Drawing for the job (mm, zero at the part's lowest x, y, z). Round coordinates to 2 decimals unless told otherwise and drop trailing zeros. Write each loop counter-clockwise with the first axis right and the second up, starting at its lowest first coordinate (ties: lowest second). Pieces come first, ordered by that corner, then holes.
Item 1: Wall check: probe 1 along X at (y, z) = (170, 3); probe 2 along Y at (x, z) = (5, 2.1). Give the ranges that are in metal, low to high.
Item 2: Band-saw the part on B-B, the plane x = 5. Write the cut outline in (y, z).
Item 3: Band-saw the part on A-A, the plane y = 5. Write the cut outline in (x, z), then the cut area to 3 significant figures.
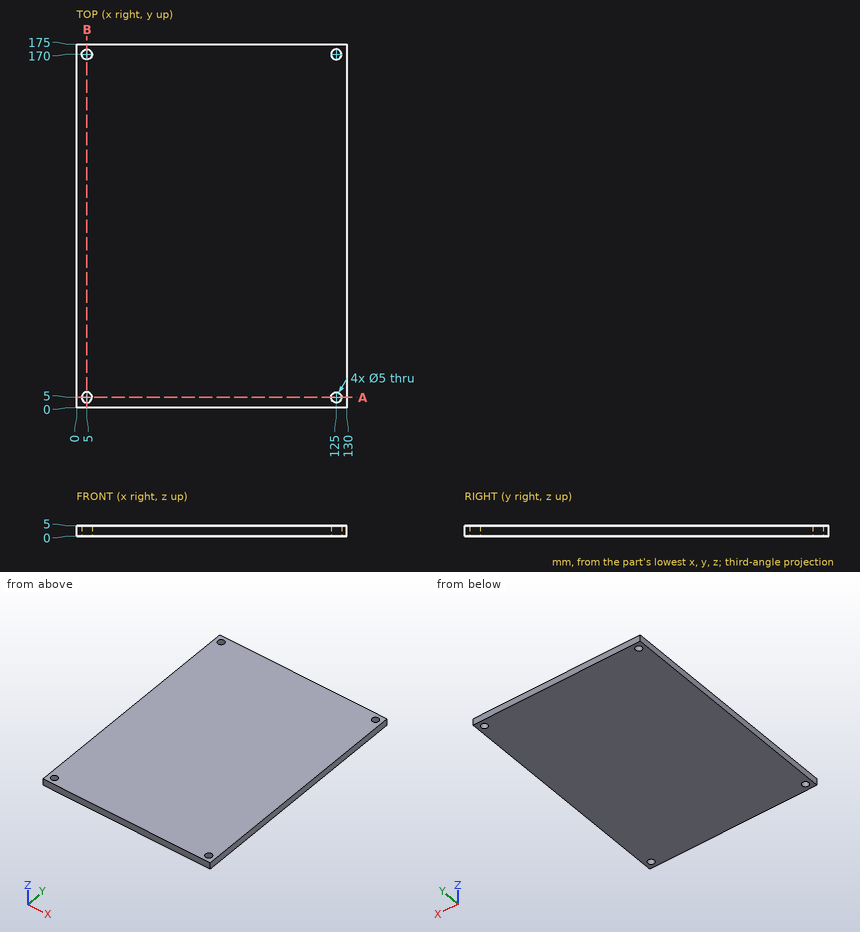
Results:
1. probe 1: x = 0 to 2.5, 7.5 to 122.5, 127.5 to 130
1. probe 2: y = 0 to 2.5, 7.5 to 167.5, 172.5 to 175
2. outline: (0, 0) - (2.5, 0) - (2.5, 5) - (0, 5) - close; (7.5, 0) - (167.5, 0) - (167.5, 5) - (7.5, 5) - close; (172.5, 0) - (175, 0) - (175, 5) - (172.5, 5) - close
3. outline: (0, 0) - (2.5, 0) - (2.5, 5) - (0, 5) - close; (7.5, 0) - (122.5, 0) - (122.5, 5) - (7.5, 5) - close; (127.5, 0) - (130, 0) - (130, 5) - (127.5, 5) - close
3. area: 600 mm2
